Read the model definition and answer for the solid it produces. Units are mm, in the model's axes. Give positions to 0.01 mm unless a question says otherwise; leave off trailing zeros. Order: outer loops, then holes, each group sorted by start corner. A loop starts at its lowest first (then second) coordinate and runs counter-clockwise, first axis right, second up. Notation, with made-up numbers: (43.25, 27.25) -> (67.25, 27.25) arc R17 cw to (67.25, 54.25) -> close; hole circle Ø11 at (24.25, -30.75). An arc over 180 degrees is marked (long way). Answer as CSV lines item,"result". Start each with the question number.
1) Flat-ended cylindrical pins translate along their axes: pin 1 Ø2.5 at (x, y) = (-7, -7) entering from -Z; pin 2 Ø2 at (x, z) = (-1.5, 153) entering from +Y. Find the tip coordinate at first contact, or state that the pin passes through.
2) Straight lines are drawn through the part: L1, parallel to Y at x = 7.25, z = 52; L2, parallel to X at y = 5.5, z = 133. For each, find the intervals that lie inside material, in ascending order. Write a range as from..to.
3) Find section C-C (z = 72). State how many separate pieces and enclosed holes the cut face has, and give its area (3 significant figures).
4) Find section A-A (y = -7). Determine the outline of the cut face in (x, z).
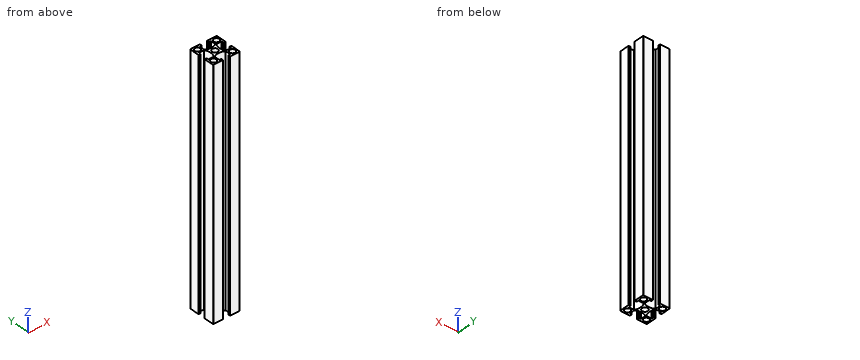
```python
from build123d import *

# Parameters (mm, degrees)
SKETCH_1_W               = 20
SKETCH_1_H               = 20
SKETCH_1_R               = 2
SKETCH_1_R_2             = 2.15
EXTRUDE_1_DEPTH          = 181
CUT_EXTRUDE_1_REACH      = 183.552
PATTERN_CIRCULAR_1_COUNT = 4
FILLET_1_R               = 0.3
SKETCH_2_R               = 2.5
CUT_EXTRUDE_2_DEPTH      = 183.375985261


with BuildPart() as part:
    # Sketch 1 → Extrude 1 (new body)
    with BuildSketch(Plane.XY):
        Rectangle(SKETCH_1_W, SKETCH_1_H)
        with Locations((-7, 7)):
            Circle(SKETCH_1_R, mode=Mode.SUBTRACT)
        with Locations((-7, -7)):
            Circle(SKETCH_1_R, mode=Mode.SUBTRACT)
        Circle(SKETCH_1_R_2, mode=Mode.SUBTRACT)
        with Locations((7, 7)):
            Circle(SKETCH_1_R, mode=Mode.SUBTRACT)
        with Locations((7, -7)):
            Circle(SKETCH_1_R, mode=Mode.SUBTRACT)
    extrude(amount=EXTRUDE_1_DEPTH)

    # Sketch 1_3 → Cut-Extrude 1 (cut, up to next)
    with BuildSketch(Plane.XY, mode=Mode.PRIVATE) as cut_extrude_1_sk1:
        with BuildLine():
            Line((-8.5, 2.65), (-10, 2.65))
            Line((-10, 2.65), (-10, -2.65))
            Line((-10, -2.65), (-8.5, -2.65))
            Line((-8.5, -2.65), (-8.5, -4.15))
            Line((-8.5, -4.15), (-4.503166667, -4.15))
            ThreePointArc((-4.503166667, -4.15), (-3.3, 0), (-4.503166667, 4.15))
            Line((-4.503166667, 4.15), (-8.5, 4.15))
            Line((-8.5, 4.15), (-8.5, 2.65))
        make_face()
    cut_extrude_1_tool1 = extrude(cut_extrude_1_sk1.sketch, amount=CUT_EXTRUDE_1_REACH, mode=Mode.PRIVATE) & part.part
    cut_extrude_1 = cut_extrude_1_tool1.solids().sort_by_distance((-6.606913, 0, 0))[0]
    add(cut_extrude_1, mode=Mode.SUBTRACT)

    # Pattern Circular 1: Cut-Extrude 1 ×4 about axis
    pattern_circular_1_axis = Axis((0, 0, 0), (0, 0, 1))
    for i in range(1, PATTERN_CIRCULAR_1_COUNT):
        add(cut_extrude_1.rotate(pattern_circular_1_axis, i * 360 / PATTERN_CIRCULAR_1_COUNT), mode=Mode.SUBTRACT)

    # Fillet 1
    fillet_1_edges = [part.edges().sort_by_distance(p)[0] for p in [
        (-10, -10, 90.5),
        (10, -10, 90.5),
        (10, 10, 90.5),
        (-10, 10, 90.5),
    ]]
    fillet(fillet_1_edges, radius=FILLET_1_R)

    # Sketch 2 → Cut-Extrude 2 (cut, through all)
    with BuildSketch(Plane.ZY.offset(10)):
        with Locations((11, 0)):
            Circle(SKETCH_2_R)
        with Locations((172, 0)):
            Circle(SKETCH_2_R)
    extrude(amount=-CUT_EXTRUDE_2_DEPTH, mode=Mode.SUBTRACT)


solid = part.part
```
Findings below:
1,pin 1,"through"
1,pin 2,"y = 3.71"
2,L1,"-10..-8.98, -5.02..-4.15, 4.15..5.02, 8.98..10"
2,L2,"-10..-8.32, -5.68..-4.15, 4.15..5.68, 8.32..10"
3,separate pieces,"1"
3,enclosed holes,"5"
3,area,"144 mm²"
4,outline,"(-10, 0) -> (-9, 0) -> (-9, 181) -> (-10, 181) -> close; (-5, 0) -> (-4.15, 0) -> (-4.15, 181) -> (-5, 181) -> close; (4.15, 0) -> (5, 0) -> (5, 181) -> (4.15, 181) -> close; (9, 0) -> (10, 0) -> (10, 181) -> (9, 181) -> close"
